CAD build for the part. Positions are in the model's coordinates, mm. A direction names the side the tool comes from. Give positions to 0.01 mm unless a question says otherwise; leave off trailing zeros. Write each loop counter-clockwise with the first axis right and the second up, starting at its lowest first coordinate (ties: lowest second). Pieces come first, ordered by that corner, then holes. Notation, with made-up numbers: (71, 83) - (106, 83) arc R9 cw to (106, 93) - close; hole circle Ø1 at (52.25, 76.25). An arc over 180 degrees is marked (long way). Put each result on its own line as item: value. Start each with the question number.
1. Cut at C-C on z = -3.4. Give the number of separate pieces and of enclosed holes in the cut face, and give its area (3 significant figures).
2. Mould opens along X. For faces 3 (the cylindrical face through (-61.32, 33.36, -2.46)), 4 (the cylindrical face through (40.552, 9.935, -2.465)), 5 (the flat face through (50, -5.14, -2)), 6 (the flat face through (-2, -10, 0)) say: +X half, -X half, draft (parallel to the pull), parting line (faces both ways), or undercut.
3. Tool access for faces 1 (the flat face through (-62.749, -11, -2)), 2 (the flat face through (-55, -15.14, -2)): list every direction of +Z, -Z, +X, -X, +Y, -Y with a clear straight run to the whole face (end or side of a thin tool).
4. Wall check: line 1 (X direction, y = -13, z = -2.15); line 2 (Y direction, x = -57, z = -3.6); line 3 (X direction, y = 6, z = -4.35). Give the ranges that are in metal, low to high.
5. Drop a flat-ended pin along its axis: pin 1 (2.5 mm diameter, centred on x = -57.75, y = -50.14, fed in from +Z). Give the stop position or say it passes through.
6. Cut at B-B on x = 42. List the corners of the cut face in (y, z), and give its area (3 significant figures).
7. Cut at A-A on y = -13.5. List the corners of the cut face in (x, z).
from build123d import *

# Parameters (mm, degrees)
EXTRUDE_1_DEPTH      = 5
SKETCH_1_4_OUTSIDE_W = 152.016
SKETCH_1_4_OUTSIDE_H = 122.016
SKETCH_1_4_OUTSIDE_R = 1.7
CUT_EXTRUDE_3_DEPTH  = 84.683501662
SKETCH_3_W           = 5
SKETCH_3_H           = 10
CUT_EXTRUDE_4_DEPTH  = 10


with BuildPart() as part:
    # 스케치1 → 보스-돌출1 (new body)
    with BuildSketch(Plane.XY):
        with BuildLine():
            Line((-57.749377558, 34.859778143), (52.250622442, 34.859778143))
            ThreePointArc((52.250622442, 34.859778143), (55.786156348, 33.395312049), (57.250622442, 29.859778143))
            Line((57.250622442, 29.859778143), (57.250622442, -50.140221857))
            ThreePointArc((57.250622442, -50.140221857), (55.786156348, -53.675755763), (52.250622442, -55.140221857))
            Line((52.250622442, -55.140221857), (-57.749377558, -55.140221857))
            ThreePointArc((-57.749377558, -55.140221857), (-61.284911464, -53.675755763), (-62.749377558, -50.140221857))
            Line((-62.749377558, -50.140221857), (-62.749377558, 29.859778143))
            ThreePointArc((-62.749377558, 29.859778143), (-61.284911464, 33.395312049), (-57.749377558, 34.859778143))
        make_face()
    extrude(amount=-EXTRUDE_1_DEPTH)

    # 스케치1<4> outside → 컷-돌출3 (cut, through all)
    # profile 1 of 9: a face of its own
    with BuildSketch(Plane.XY):
        with Locations((-2.749, -10.14)):
            Rectangle(SKETCH_1_4_OUTSIDE_W, SKETCH_1_4_OUTSIDE_H)
        with BuildLine():
            Line((-57.749377558, 34.859778143), (52.250622442, 34.859778143))
            ThreePointArc((52.250622442, 34.859778143), (55.786156348, 33.395312049), (57.250622442, 29.859778143))
            Line((57.250622442, 29.859778143), (57.250622442, -50.140221857))
            ThreePointArc((57.250622442, -50.140221857), (55.786156348, -53.675755763), (52.250622442, -55.140221857))
            Line((52.250622442, -55.140221857), (-57.749377558, -55.140221857))
            ThreePointArc((-57.749377558, -55.140221857), (-61.284911464, -53.675755763), (-62.749377558, -50.140221857))
            Line((-62.749377558, -50.140221857), (-62.749377558, 29.859778143))
            ThreePointArc((-62.749377558, 29.859778143), (-61.284911464, 33.395312049), (-57.749377558, 34.859778143))
        make_face(mode=Mode.SUBTRACT)
    # profile 2 of 9: a face of its own
    with BuildSketch(Plane.XY):
        with Locations((-57.749377558, 29.859778143)):
            Circle(SKETCH_1_4_OUTSIDE_R)
    # profile 3 of 9: a face of its own
    with BuildSketch(Plane.XY):
        with Locations((52.250622442, 29.859778143)):
            Circle(SKETCH_1_4_OUTSIDE_R)
    # profile 4 of 9: a face of its own
    with BuildSketch(Plane.XY):
        with Locations((-57.749377558, -50.140221857)):
            Circle(SKETCH_1_4_OUTSIDE_R)
    # profile 5 of 9: a face of its own
    with BuildSketch(Plane.XY):
        with Locations((52.250622442, -50.140221857)):
            Circle(SKETCH_1_4_OUTSIDE_R)
    # profile 6 of 9: a face of its own
    with BuildSketch(Plane.XY):
        with Locations((-47.749377558, 9.859778143)):
            Circle(SKETCH_1_4_OUTSIDE_R)
    # profile 7 of 9: a face of its own
    with BuildSketch(Plane.XY):
        with Locations((-47.749377558, -30.140221857)):
            Circle(SKETCH_1_4_OUTSIDE_R)
    # profile 8 of 9: a face of its own
    with BuildSketch(Plane.XY):
        with Locations((42.250622442, 9.859778143)):
            Circle(SKETCH_1_4_OUTSIDE_R)
    # profile 9 of 9: a face of its own
    with BuildSketch(Plane.XY):
        with Locations((42.250622442, -30.140221857)):
            Circle(SKETCH_1_4_OUTSIDE_R)
    extrude(amount=-CUT_EXTRUDE_3_DEPTH, mode=Mode.SUBTRACT)

    # 스케치3 → 컷-돌출4 (cut)
    with BuildSketch(Plane.XY):
        with Locations((-55.249377558, -10.140221857)):
            Rectangle(SKETCH_3_W, SKETCH_3_H)
        with Locations((49.750622442, -10.140221857)):
            Rectangle(SKETCH_3_W, SKETCH_3_H)
        with Locations((-55.249377558, 9.881604628)):
            Rectangle(SKETCH_3_W, SKETCH_3_H)
    extrude(amount=-CUT_EXTRUDE_4_DEPTH, mode=Mode.SUBTRACT)


solid = part.part
Report:
1. separate pieces: 1
1. enclosed holes: 11
1. area: 10,600 mm²
2. face 3: -X half
2. face 4: undercut
2. face 5: undercut
2. face 6: draft
3. face 1: +Z, -Z, -X, +Y, -Y
3. face 2: +Z, -Z
4. line 1: x = -62.75 to -57.75, -52.75 to 47.25, 52.25 to 57.25
4. line 2: y = -55.14 to -51.67, -48.61 to -15.14, -5.14 to 4.88, 14.88 to 28.33, 31.39 to 34.86
4. line 3: x = -62.75 to -57.75, -52.75 to 57.25
5. pin 1: passes through
6. outline: (-55.14, -5) - (-31.82, -5) - (-31.82, 0) - (-55.14, 0) - close; (-28.46, -5) - (8.18, -5) - (8.18, 0) - (-28.46, 0) - close; (11.54, -5) - (34.86, -5) - (34.86, 0) - (11.54, 0) - close
6. area: 416 mm²
7. outline: (-62.75, -5) - (-57.75, -5) - (-57.75, 0) - (-62.75, 0) - close; (-52.75, -5) - (47.25, -5) - (47.25, 0) - (-52.75, 0) - close; (52.25, -5) - (57.25, -5) - (57.25, 0) - (52.25, 0) - close
